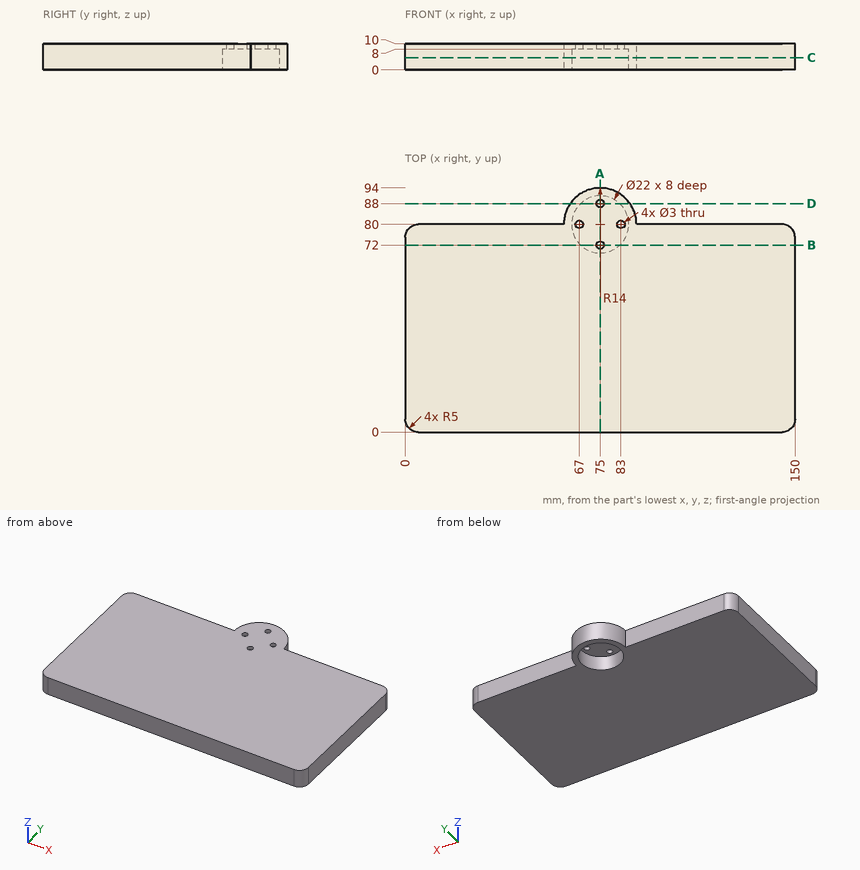
Print and shaded views of the part. All mm, measured from the part's lowest x, y and z. Coordinates: 2 decimals unless noted, no trailing zeros. Write each loop counter-clockwise with the first axis right and the second up, starting at its lowest first coordinate (ties: lowest second). Pieces come first, ordered by that corner, then holes.
(1) Drill centre lines: probe 1 along Y at (x, z) = (75, 8.45); probe 2 along X at (y, z) = (72, 8.95); probe 3 along Y at (x, z) = (74.5, 1). Where is each one in solid material? Low to high.
(2) Cut at A-A, the plane x = 75. List the corners of the cut face in (y, z).
(3) Cut at D-D, the plane y = 88. List the corners of the cut face in (x, z), and give its area (3 significant figures).
(4) Cut at C-C, the plane z = 4.75. List the corners of the cut face in (x, y), and give its area (3 significant figures).
(5) Cut at B-B, the plane y = 72. List the corners of the cut face in (x, z).
(6) Flat gauge pins, fed straight in: pin 1 (3.5 mm diameter, centred on x = 75, y = 88, fed in from -Z); pin 2 (1 mm diameter, centred on y = 83, z = 2, fed in from -X) (3 decimals); pin 3 (3 mm diameter, centred on x = 112, z = 4, fed in from +Y). Where does each tip first touch, or does it go through?
Geometry says:
1. probe 1: y = 0 to 70.5, 73.5 to 86.5, 89.5 to 94
1. probe 2: x = 0 to 73.5, 76.5 to 150
1. probe 3: y = 0 to 69.01, 90.99 to 93.99
2. outline: (0, 0) - (69, 0) - (69, 8) - (70.5, 8) - (70.5, 10) - (0, 10) - close; (73.5, 8) - (86.5, 8) - (86.5, 10) - (73.5, 10) - close; (89.5, 8) - (91, 8) - (91, 0) - (94, 0) - (94, 10) - (89.5, 10) - close
3. outline: (63.51, 0) - (67.45, 0) - (67.45, 8) - (73.5, 8) - (73.5, 10) - (63.51, 10) - close; (76.5, 8) - (82.55, 8) - (82.55, 0) - (86.49, 0) - (86.49, 10) - (76.5, 10) - close
3. area: 103 mm2
4. outline: (0, 5) arc R5 ccw to (5, 0) - (145, 0) arc R5 ccw to (150, 5) - (150, 75) arc R5 ccw to (145, 80) - (89, 80) arc R14 ccw to (61, 80) - (5, 80) arc R5 ccw to (0, 75) - close; hole circle Ø22 at (75, 80)
4. area: 11,900 mm2
5. outline: (0, 0) - (67.45, 0) - (67.45, 8) - (73.5, 8) - (73.5, 10) - (0, 10) - close; (76.5, 8) - (82.55, 8) - (82.55, 0) - (150, 0) - (150, 10) - (76.5, 10) - close
6. pin 1: stops at z = 8
6. pin 2: stops at x = 61.225
6. pin 3: stops at y = 80
